Autodesk Inventor part; units mm, degrees
ref_plane "Work Plane1" through (0, 0, 20.4) normal (0, 0, 1) x (1, 0, 0)
ref_plane "YZ Plane" through (0, 0, 0) normal (1, 0, 0) x (0, 1, 0)
ref_plane "XZ Plane" through (0, 0, 0) normal (0, 1, 0) x (-1, 0, 0)
sketch "Sketch1" plane through (0, 0, 0) normal (0, 0, 1) x (1, 0, 0)
  line L0 (-25, -5.5) -> (25, -5.5)
  line L1 (25, -5.5) -> (25, 5.5)
  line L2 (25, 5.5) -> (-25, 5.5)
  line L3 (-25, 5.5) -> (-25, -5.5)
  line L4 (-25, -5.5) -> (25, 5.5) construction
  line L5 (25, -5.5) -> (-25, 5.5) construction
  point P0 (0, 0)
  dimension "d0" = 50
  dimension "d1" = 11
extrude "Extrusion1" add sketch "Sketch1" along normal mid plane 0.8
sketch "Sketch2" plane through (0, 0, 0.4) normal (0, 0, 1) x (1, 0, 0)
  line L0 (25, 5.5) -> (-25, 5.5)
  line L1 (-25, -5.5) -> (25, -5.5)
  line L2 (-25, 5.5) -> (-10, 5.5)
  line L3 (-10, 5.5) -> (-10, -5.5)
  line L4 (-10, -5.5) -> (-25, -5.5)
  line L5 (-25, -5.5) -> (-25, 5.5)
  point P0 (0, 0)
  dimension "d4" = 15
  dimension "d5" = 11
extrude "Extrusion2" add sketch "Sketch2" along normal blind 0.2
sketch "Sketch3" plane through (0, 0, 0.6) normal (0, 0, 1) x (1, 0, 0)
  line L0 (-25, 4.25) -> (-10, 4.25)
  line L1 (-10, 4.25) -> (-10, 3.25)
  line L2 (-10, 3.25) -> (-25, 3.25)
  line L3 (-25, 3.25) -> (-25, 4.25)
  line L4 (-25, 5.5) -> (-25, -5.5)
  line L5 (-10, 5.5) -> (-25, 5.5)
  line L6 (-10, 0.75) -> (-25, 0.75)
  line L7 (-10, 1.75) -> (-10, 0.75)
  line L8 (-25, 1.75) -> (-10, 1.75)
  line L9 (-25, 0.75) -> (-25, 1.75)
  line L10 (-10, -1.75) -> (-25, -1.75)
  line L11 (-10, -0.75) -> (-10, -1.75)
  line L12 (-25, -0.75) -> (-10, -0.75)
  line L13 (-25, -1.75) -> (-25, -0.75)
  line L14 (-10, -4.25) -> (-25, -4.25)
  line L15 (-10, -3.25) -> (-10, -4.25)
  line L16 (-25, -3.25) -> (-10, -3.25)
  line L17 (-25, -4.25) -> (-25, -3.25)
  point P0 (0, 0)
  dimension "d8" = 15
  dimension "d9" = 1
  dimension "d10" = 1.25
  dimension "d13" = 2.5
extrude "Extrusion3" cut sketch "Sketch3" against normal blind 0.5
ref_plane "Work Plane1" through (0, 0, 20.4) normal (0, 0, 1) x (1, 0, 0)
sketch "Sketch4" plane through (0, 0, 20.4) normal (0, 0, 1) x (1, 0, 0)
  line L0 (-10, 5.5) -> (-25, 5.5)
  line L1 (-9.9335, 7.1739) -> (25.0665, 7.1739) construction
  line L2 (25.0665, 7.1739) -> (25.0665, -7.4481) construction
  line L3 (25.0665, -7.4481) -> (-9.9335, -7.4481) construction
  line L4 (-9.9335, -7.4481) -> (-9.9335, 7.1739) construction
  point P0 (0, 0)
  dimension "d56" = 35
decal "Decal1"
sketch "Sketch5" plane through (0, 0, 20.4) normal (0, 0, 1) x (1, 0, 0)
  point P0 (0, 0)
properties part number "Pen2" material "Acetal Resin, Black"
The listing builds one solid part. Answer for the finished solid, in the listing's coordinates (mm). A direction names the side the tool comes from. Give positions to 0.01 mm unless a question says otherwise; leave off trailing zeros. Order: outer loops, then holes, each group sorted by start corner. A loop starts at its lowest first (then second) coordinate and runs counter-clockwise, first axis right, second up. Notation, with made-up numbers: (82.5, -36) - (88.5, -36) arc R22 cw to (88.5, -25) - close; hole circle Ø2 at (-29, -27). An arc over 180 degrees is marked (long way). Answer in a Markdown table with one row per item. Add a question column.
Q1. The part is cut by section A-A (y = 2.75). Determine the outline of the cut face in (x, z), then the cut area to 3 significant figures.
Q2. Find the intervals of material crossed by line 1 along Y through (x, z) = (-15.5, 0.55); line 2 along X through (y, z) = (2, 0.5); line 3 along Z through (x, y) = (11.5, 1.25), in increasing order. Write a range as [from, to].
Q3. Given P1, Ø3.5, axis at x = 3, y = 1.5, coming from the +Z side, flat-ended and moving along its own axis, determine where the tip first touches the part or whether it passes through.
Q4. The part is cut by section B-B (x = -13.5). Determine the outline of the cut face in (y, z), then the cut area to 3 significant figures.
Q5. Which of the six approach directions +Z, -Z, +X, -X, +Y, -Y give full straight-line access (tool end or side, diameter ignored) to faces 5 (the flat face through (-18, 3, 0.6)), 6 (the flat face through (-18, -4, 0.1)), 7 (the flat face through (7, 0, 0.4))?
Q6. For a pull along Y with two mould halves and no side action, classify faces 1 (the flat face through (-18, -1, 0.1)), 2 (the flat face through (-18, 4, 0.1)), 3 (the flat face through (0, -5.5, 0)), 4 (the flat face through (-18, 0, 0.6)) as released by +Y, released by -Y, zero draft, split by the parting line, or undercut.
Q7. The part is cut by section D-D (x = 0). Determine the outline of the cut face in (y, z), then the cut area to 3 significant figures.
Q8. The part is cut by section C-C (z = 0.25). Determine the outline of the cut face in (x, y), then the cut area to 3 significant figures.
Determined:
| question | item | result |
|---|---|---|
| 1 | outline | (-25, -0.4) - (25, -0.4) - (25, 0.4) - (-10, 0.4) - (-10, 0.6) - (-25, 0.6) - close |
| 1 | area | 43.0 mm² |
| 2 | line 1 | y = [-5.5, -4.25], [-3.25, -1.75], [-0.75, 0.75], [1.75, 3.25], [4.25, 5.5] |
| 2 | line 2 | x = [-25, -10] |
| 2 | line 3 | z = [-0.4, 0.4] |
| 3 | P1 | stops at z = 0.4 |
| 4 | outline | (-5.5, -0.4) - (5.5, -0.4) - (5.5, 0.6) - (4.25, 0.6) - (4.25, 0.1) - (3.25, 0.1) - (3.25, 0.6) - (1.75, 0.6) - (1.75, 0.1) - (0.75, 0.1) - (0.75, 0.6) - (-0.75, 0.6) - (-0.75, 0.1) - (-1.75, 0.1) - (-1.75, 0.6) - (-3.25, 0.6) - (-3.25, 0.1) - (-4.25, 0.1) - (-4.25, 0.6) - (-5.5, 0.6) - close |
| 4 | area | 9.00 mm² |
| 5 | face 5 | +Z, +X, -X, +Y, -Y |
| 5 | face 6 | +Z, -X |
| 5 | face 7 | +Z, +X, +Y, -Y |
| 6 | face 1 | undercut |
| 6 | face 2 | undercut |
| 6 | face 3 | released by -Y |
| 6 | face 4 | zero draft |
| 7 | outline | (-5.5, -0.4) - (5.5, -0.4) - (5.5, 0.4) - (-5.5, 0.4) - close |
| 7 | area | 8.80 mm² |
| 8 | outline | (-25, -5.5) - (25, -5.5) - (25, 5.5) - (-25, 5.5) - (-25, 4.25) - (-10, 4.25) - (-10, 3.25) - (-25, 3.25) - (-25, 1.75) - (-10, 1.75) - (-10, 0.75) - (-25, 0.75) - (-25, -0.75) - (-10, -0.75) - (-10, -1.75) - (-25, -1.75) - (-25, -3.25) - (-10, -3.25) - (-10, -4.25) - (-25, -4.25) - close |
| 8 | area | 490 mm² |
